For this review, take the finished solid that the model builds, in its own axes (mm). Face numbers are marked on the shaded views. A direction names the side the tool comes from. Coordinates: 2 decimals unless noted, no trailing zeros. Loops run counter-clockwise (first coordinate to the right, second up) from the corner with the lowest first, then second, coordinate; pieces in that order, holes last. Notation, with made-up numbers: M -2,31.5 L 54,31.5 A25 ccw 54,46.5 Z; hole C 39,-24 d2. An arc over 180 degrees is marked long. Answer as a JSON object with one key per item and string values. Group by question number.
Item 1: Mouldability with a two-part tool opening along X and no side actions: class the marked faces 4, 5, 6 and 7 as +X half, -X half, draft (parallel to the pull), parting line (faces both ways), or undercut.
Item 2: Add section A-A (y = 0). State the section outline as (x, z) points.
Item 3: Insertion check: pin 1 (3 mm diameter, centred on x = -5.5, y = -6.5, fed in from +Z); pin 2 (1.5 mm diameter, centred on x = -1, z = 0, fed in from +Y); pin 3 (3 mm diameter, centred on x = 0.5, z = -6, fed in from +Y); pin 4 (3 mm diameter, centred on x = 12.78, y = -10.2, fed in from +Z). Each pin has a flat end and moves straight along its axis. Give the tip position at first contact, or say it passes through.
Item 4: Add section D-D (x = 16). State the section outline as (y, z) points, then the cut area to 3 significant figures.
Item 5: Wall thickness on L1, parallel to Z at x = 5, y = -16; L2, parallel to X at y = 2, z = -3.5; L3, parallel to X at y = -4.5, z = 0.5: over which ranges is each line inside the solid? List them lowest first. Write a range as from..to.
Item 6: Tool access review of the marked faces 1, 2 and 3: name each direction out of +Z, -Z, +X, -X, +Y, -Y from which nothing blocks a thin tool from reaching the whole face with its end or side.
Item 7: Add section C-C (z = -2.5). State the section outline as (x, y) points, then the cut area to 3 significant figures.
Autodesk Inventor part; units mm, degrees
ref_plane "Work Plane1" through (-47.7309, -37.9502, -7.3) normal (0, 0, 1) x (0.9998, 0.0216, 0)
ref_plane "YZ Plane" through (0, 0, 0) normal (1, 0, 0) x (0, 1, 0)
ref_plane "XZ Plane" through (0, 0, 0) normal (0, 1, 0) x (-1, 0, 0)
sketch "Sketch1" plane through (0, 0, 0) normal (0, 0, 1) x (1, 0, 0)
  circle A0 centre (0, 0) radius 12.7
  circle A1 centre (0, 0) radius 10.5
  circle A2 centre (0, 0) radius 14.3
  dimension "d0" = 1.6
extrude "Extrusion1" add sketch "Sketch1" along normal blind 1.6 contours A0 | A2
sketch "Sketch2" plane through (0, 0, 0) normal (0, 0, -1) x (-1, 0, 0)
  circle A0 centre (0, 0) radius 12.7
  circle A1 centre (0, 0) radius 14.3
  circle A2 centre (0, 0) radius 13
  dimension "d3" = 0.3
extrude "Extrusion2" add sketch "Sketch2" along normal blind 6.3 contours A1
sketch "Sketch3" plane through (0, 0, -6.3) normal (0, 0, -1) x (-1, 0, 0)
  circle A0 centre (0, 0) radius 14.3
  circle A1 centre (19.8743, -0.3764) radius 0.95
  circle A2 centre (12.6657, 10.2607) radius 0.95
  circle A3 centre (-12.3285, 10.8) radius 1.05
  circle A4 centre (-20.1164, 0.4865) radius 0.95
  circle A5 centre (-12.7815, -10.1951) radius 0.95
  circle A6 centre (12.2127, -10.7344) radius 0.95
  circle A7 centre (0, 0) radius 18.8
  circle A8 centre (0, 0) radius 13
  dimension "d6" = 4.5
ref_plane "Work Plane1" through (-47.7309, -37.9502, -7.3) normal (0, 0, 1) x (0.9998, 0.0216, 0)
extrude "Extrusion3" add sketch "Sketch3" along normal up to surface (1 mm away) contours A0 | A7
fillet "Fillet1" radius 1 1 edges at (14.3, 0, -6.3)
sketch "Sketch4" plane through (0, 0, -6.3) normal (0, 0, 1) x (1, 0, 0)
  circle A0 centre (-12.2127, -10.7344) radius 0.95
  circle A1 centre (-12.2127, -10.7344) radius 2.5
  circle A2 centre (12.7815, -10.1951) radius 0.95
  circle A3 centre (12.7815, -10.1951) radius 2.5
  circle A4 centre (12.3285, 10.8) radius 1.05
  circle A5 centre (12.3285, 10.8) radius 2.5
  circle A6 centre (-12.6657, 10.2607) radius 0.95
  circle A7 centre (-12.6657, 10.2607) radius 2.5
  circle A8 centre (-12.2127, -10.7344) radius 0.95
  point P0 (0, 0)
  point P1 (-11.31, -10.3041)
  point P2 (-11.6701, -9.8944)
  dimension "d10" = 5
  dimension "d11" = 5
  dimension "d12" = 5
  dimension "d13" = 5
extrude "Extrusion4" cut sketch "Sketch4" along normal blind 8.05
properties part number "FilterHolder"
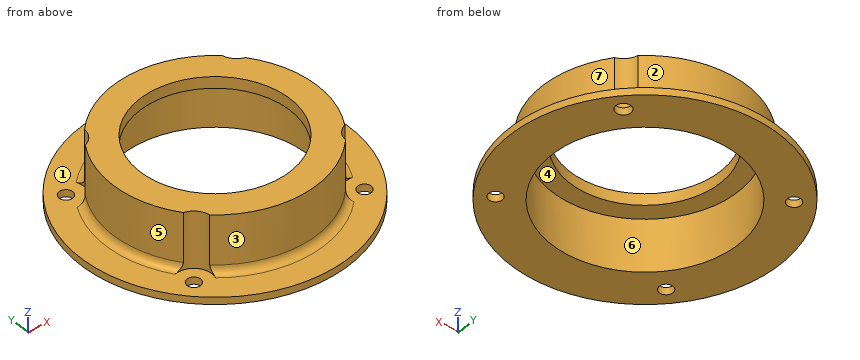
From the geometry:
{
 "1": {"face 4": "undercut", "face 5": "-X half", "face 6": "undercut", "face 7": "+X half"},
 "2": {"outline": "M -18.8,-7.3 L -13,-7.3 L -13,0 L -10.5,0 L -10.5,1.6 L -14.3,1.6 L -14.3,-5.3 A1 cw -15.3,-6.3 L -18.8,-6.3 Z; M 10.5,0 L 13,0 L 13,-7.3 L 18.8,-7.3 L 18.8,-6.3 L 15.3,-6.3 A1 cw 14.3,-5.3 L 14.3,1.6 L 10.5,1.6 Z"},
 "3": {"pin 1": "passes through", "pin 2": "stops at y = 14.3", "pin 3": "stops at y = 18.8", "pin 4": "stops at z = -6.3"},
 "4": {"outline": "M -9.87,-7.3 L 9.87,-7.3 L 9.87,-6.3 L -9.87,-6.3 Z", "area": "19.7 mm²"},
 "5": {"L1": "z = -7.3..-6.3", "L2": "x = -14.16..-12.85, 12.85..14.16", "L3": "x = -13.57..-9.49, 9.49..13.57"},
 "6": {"face 1": "+Z", "face 2": "+Z, +Y", "face 3": "+Z, -Y"},
 "7": {"outline": "M -11.94,7.87 A14.3 ccw -11.64,-8.3 A2.5 cw -9.73,-10.48 A14.3 ccw 10.3,-9.92 A2.5 cw 11.96,-7.83 A14.3 ccw 11.56,8.42 A2.5 cw 9.87,10.35 A14.3 ccw -10.17,10.05 A2.5 cw Z; hole C 0,0 d26", "area": "108 mm²"}
}
